from build123d import *

# Parameters (mm, degrees)
BOSS_EXTRUDE1_DEPTH = 43
CUT_EXTRUDE1_START  = -6
SKETCH3_W           = 51
SKETCH3_H           = 4
CUT_EXTRUDE1_DEPTH  = 31
CUT_EXTRUDE2_REACH  = 74.18
SKETCH4_W           = 20
SKETCH4_H           = 20
BOSS_EXTRUDE2_START = -21
BOSS_EXTRUDE2_DEPTH = 30
CUT_EXTRUDE3_REACH  = 74.18
SKETCH6_W           = 5
SKETCH6_H           = 7.3


with BuildPart() as part:
    # Sketch1 → Boss-Extrude1 (new body)
    with BuildSketch(Plane.XY):
        Polygon((1, 15), (5, 15), (5, 4), (56, 4), (56, -3.3), (1, -3.3), align=None)
    extrude(amount=BOSS_EXTRUDE1_DEPTH)

    # Sketch3 → Cut-Extrude1 (cut)
    with BuildSketch(Plane.XY.offset(43).offset(CUT_EXTRUDE1_START)):
        with Locations((30.5, 2)):
            Rectangle(SKETCH3_W, SKETCH3_H)
    extrude(amount=-CUT_EXTRUDE1_DEPTH, mode=Mode.SUBTRACT)

    # Sketch4 → Cut-Extrude2 (cut, up to next)
    with BuildSketch(Plane(origin=(0, 0, 0), x_dir=(1, 0, 0), z_dir=(0, 1, 0)), mode=Mode.PRIVATE) as cut_extrude2_sk1:
        with Locations((23.57, -21.5)):
            Rectangle(SKETCH4_W, SKETCH4_H)
    cut_extrude2_tool1 = extrude(cut_extrude2_sk1.sketch, amount=-CUT_EXTRUDE2_REACH, mode=Mode.PRIVATE) & part.part
    add(cut_extrude2_tool1.solids().sort_by_distance((23.57, 0, 21.5))[0], mode=Mode.SUBTRACT)

    # Sketch5 → Boss-Extrude2 (add)
    with BuildSketch(Plane(origin=(56, 0, 0), x_dir=(0, 0, -1), z_dir=(1, 0, 0)).offset(BOSS_EXTRUDE2_START)):
        Polygon((-6, 7), (-6, 4), (0, 4), (0, 7), (-2.5, 7), (-2.5, 12), (0, 12), (0, 15), (-6, 15), (-6, 12), (-3.5, 12), (-3.5, 7), align=None)
        Polygon((-37, 4), (-37, 7), (-39.5, 7), (-39.5, 12), (-37, 12), (-37, 15), (-43, 15), (-43, 12), (-40.5, 12), (-40.5, 7), (-43, 7), (-43, 4), align=None)
    extrude(amount=-BOSS_EXTRUDE2_DEPTH)

    # Sketch6 → Cut-Extrude3 (cut, up to next)
    with BuildSketch(Plane(origin=(0, 0, 0), x_dir=(-1, 0, 0), z_dir=(0, 0, -1)), mode=Mode.PRIVATE) as cut_extrude3_sk1:
        with Locations((-53.5, 0.35)):
            Rectangle(SKETCH6_W, SKETCH6_H)
    cut_extrude3_tool1 = extrude(cut_extrude3_sk1.sketch, amount=-CUT_EXTRUDE3_REACH, mode=Mode.PRIVATE) & part.part
    add(cut_extrude3_tool1.solids().sort_by_distance((53.5, 0.35, 0))[0], mode=Mode.SUBTRACT)


solid = part.part
Design review of the part built by this model. Coordinates are the model's own, in mm. A direction names the side the tool comes from. Coordinates: 2 decimals unless noted, no trailing zeros. Order: outer loops, then holes, each group sorted by start corner. A loop starts at its lowest first (then second) coordinate and runs counter-clockwise, first axis right, second up.
Item 1: Take a section at C-C, the plane z = 23. Write out the cut boundary in (x, y), then the cut area to 3 significant figures.
Item 2: Take a section at D-D, the plane x = 6. Write out the cut boundary in (y, z).
Item 3: For line 1 (Z direction, x = 34.5, y = 8); line 2 (Z direction, x = 6, y = 5.75); line 3 (X direction, y = 0.75, z = 29), list the stretches that pass through material, from the lowest coordinate up.
Item 4: For pin 1 Ø5 at (y, z) = (7.5, 40.5) entering from +X; pin 2 Ø1 at (y, z) = (4.5, 10) entering from +X; pin 3 Ø4 at (x, y) = (26, 9.5) entering from -Z, all flat-tipped, find the tip position at first contact; note any pin that passes through.
Item 5: For faces 4 (the flat face through (20, 7, 42)), 5 (the flat face through (23, -2, 31.5)), 6 (the flat face through (23, 4, 6)), 7 (the flat face through (20, 7, 38)), 8 (the flat face through (20, 12, 1)), list the 3-axis set-ups (+Z, -Z, +X, -X, +Y, -Y) from which the entire face can be reached by the end or side of a thin tool; tool diameter is ignored.
Item 6: The part is to be moulded in two halves that separate along Y. For faces 1 (the flat face through (20, 9, 39.5)), 2 (the flat face through (33.57, -2, 22)), 3 (the flat face through (43, 4, 40)), say which applies: pulls with the +Y half, pulls with the -Y half, needs draft (parallel to the pull), parting line crosses it, or undercut.
Item 7: Take a section at B-B, the plane y = -1.75. Write out the cut boundary in (x, z), then the cut area to 3 significant figures.
Item 8: Take a section at A-A, the plane x = 24. Write out the cut boundary in (y, z), then the cut area to 3 significant figures.
The answers:
1. outline: (1, -3.3) - (13.57, -3.3) - (13.57, 0) - (5, 0) - (5, 15) - (1, 15) - close; (33.57, -3.3) - (51, -3.3) - (51, 0) - (33.57, 0) - close
1. area: 159 mm2
2. outline: (-3.3, 0) - (7, 0) - (7, 2.5) - (12, 2.5) - (12, 0) - (15, 0) - (15, 6) - (12, 6) - (12, 3.5) - (7, 3.5) - (7, 6) - (0, 6) - (0, 37) - (7, 37) - (7, 39.5) - (12, 39.5) - (12, 37) - (15, 37) - (15, 43) - (12, 43) - (12, 40.5) - (7, 40.5) - (7, 43) - (-3.3, 43) - close
3. line 1: z = 2.5 to 3.5, 39.5 to 40.5
3. line 2: z = 0 to 6, 37 to 43
3. line 3: x = 1 to 5
4. pin 1: stops at x = 35
4. pin 2: stops at x = 5
4. pin 3: stops at z = 2.5
5. face 4: +Z, +X
5. face 5: +Y, -Y
5. face 6: +X, +Y
5. face 7: +X
5. face 8: -Z, +X
6. face 1: undercut
6. face 2: needs draft
6. face 3: pulls with the +Y half
7. outline: (1, 0) - (51, 0) - (51, 43) - (1, 43) - close; hole (13.57, 11.5) - (33.57, 11.5) - (33.57, 31.5) - (13.57, 31.5) - close
7. area: 1,750 mm2
8. outline: (-3.3, 0) - (7, 0) - (7, 2.5) - (12, 2.5) - (12, 0) - (15, 0) - (15, 6) - (12, 6) - (12, 3.5) - (7, 3.5) - (7, 6) - (0, 6) - (0, 11.5) - (-3.3, 11.5) - close; (-3.3, 31.5) - (0, 31.5) - (0, 37) - (7, 37) - (7, 39.5) - (12, 39.5) - (12, 37) - (15, 37) - (15, 43) - (12, 43) - (12, 40.5) - (7, 40.5) - (7, 43) - (-3.3, 43) - close
8. area: 206 mm2
